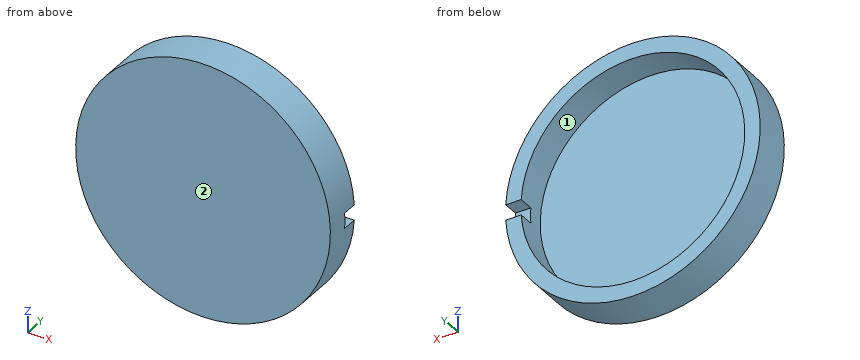
```python
from build123d import *

# Parameters (mm, degrees)
SKETCH_2_W          = 2.034523859
SKETCH_2_H          = 2
CUT_EXTRUDE_1_DEPTH = 2


with BuildPart() as part:
    # Эскиз1 → Повернуть1 (revolve)
    with BuildSketch(Plane(origin=(0, 0, 0), x_dir=(0, 0, -1), z_dir=(1, 0, 0))):
        Polygon((0, 0), (16.5, 0), (16.5, 5), (14.5, 5), (14.5, 1), (0, 1), align=None)
    revolve(axis=Axis((0, 1, 0), (0, -1, 0)))

    # Эскиз2 → Вырез-Вытянуть1 (cut)
    with BuildSketch(Plane(origin=(0, 5, 0), x_dir=(1, 0, 0), z_dir=(0, 1, 0))):
        with Locations((15.482738071, 0)):
            Rectangle(SKETCH_2_W, SKETCH_2_H)
    extrude(amount=-CUT_EXTRUDE_1_DEPTH, mode=Mode.SUBTRACT)


solid = part.part
```
Build history of the part. All positions in model axes, mm. Face numbers are marked on the shaded views. A direction names the side the tool comes from. Round coordinates to 2 decimals unless told otherwise and drop trailing zeros. Loops run counter-clockwise (first coordinate to the right, second up) from the corner with the lowest first, then second, coordinate; pieces in that order, holes last.
Item 1: Saw through at A-A (z = 0). List the corners of the cut face in (x, y).
Item 2: Drill centre lines: line 1 along Z through (x, y) = (0, 4.15); line 2 along Y through (x, z) = (6, 3); line 3 along Z through (x, y) = (-10, 3.1). Where is each one in solid material? Low to high.
Item 3: Saw through at B-B (x = 0). List the corners of the cut face in (y, z).
Item 4: Saw through at C-C (y = 1.95). List the corners of the cut face in (x, z), then the cut area to 3 significant figures.
Item 5: Pin check, flat tips, straight feed: P1, Ø3, axis at y = 3, z = -11.5, coming from the +X side; P2, Ø2, axis at x = 16, y = 4.5, coming from the +Z side; P3, Ø1, axis at x = 15.5, y = 4, coming from the -Z side. Stop position of each tip, or through.
Item 6: Which spindle directions (+Z, -Z, +X, -X, +Y, -Y) get a long thin tool onto all of the face, cutting with end or side? Do the marked faces 1 and 2. Say none if no direction does.
Worked answers:
1. outline: (-16.5, 0) - (16.5, 0) - (16.5, 3) - (14.5, 3) - (14.5, 1) - (-14.5, 1) - (-14.5, 5) - (-16.5, 5) - close
2. line 1: z = -16.5 to -14.5, 14.5 to 16.5
2. line 2: y = 0 to 1
2. line 3: z = -13.12 to -10.5, 10.5 to 13.12
3. outline: (0, -16.5) - (5, -16.5) - (5, -14.5) - (1, -14.5) - (1, 14.5) - (5, 14.5) - (5, 16.5) - (0, 16.5) - close
4. outline: circle Ø33 at (0, 0); hole circle Ø29 at (0, 0)
4. area: 195 mm2
5. P1: stops at x = 13.12
5. P2: stops at z = 6.87
5. P3: stops at z = -6.87
6. face 1: +Y
6. face 2: +Z, -Z, +X, -X, -Y
